Build history of the part. All positions in model axes, mm. A direction names the side the tool comes from. Give positions to 0.01 mm unless a question says otherwise; leave off trailing zeros. Order: outer loops, then holes, each group sorted by start corner. A loop starts at its lowest first (then second) coordinate and runs counter-clockwise, first axis right, second up. Notation, with made-up numbers: (10, 33.25) - (39, 33.25) arc R33 cw to (39, 68.25) - close; hole circle Ø4 at (51, 17.5). An arc over 180 degrees is marked (long way). Use a Markdown table: item, result.
from build123d import *

# Parameters (mm, degrees)
BASE_FLANGE1_DEPTH      = 45
EDGE_FLANGE1_DEPTH      = 606
EDGE_FLANGE1_BEND_DEPTH = 606
SKETCH11_R              = 12
CUT_EXTRUDE1_DEPTH      = 10
FILLET1_R               = 3
M5_CLEARANCE_HOLE1_D    = 5.8
M5_CLEARANCE_HOLE2_D    = 5.8


# Sheet-metal steps are written as plain solids
with BuildPart() as part:
    # Sketch1 → Base-Flange1 (new, symmetric)
    with BuildSketch(Plane.XY):
        with BuildLine():
            Line((-325, 0), (-309, 0))
            ThreePointArc((-309, 0), (-306.171572875, 1.171572875), (-305, 4))
            Line((-305, 4), (-305, 48))
            ThreePointArc((-305, 48), (-304.414213562, 49.414213562), (-303, 50))
            Line((-303, 50), (303, 50))
            ThreePointArc((303, 50), (304.414213562, 49.414213562), (305, 48))
            Line((305, 48), (305, 4))
            ThreePointArc((305, 4), (306.171572875, 1.171572875), (309, 0))
            Line((309, 0), (325, 0))
            Line((325, 0), (325, 2))
            Line((325, 2), (309, 2))
            ThreePointArc((309, 2), (307.585786438, 2.585786438), (307, 4))
            Line((307, 4), (307, 48))
            ThreePointArc((307, 48), (305.828427125, 50.828427125), (303, 52))
            Line((303, 52), (-303, 52))
            ThreePointArc((-303, 52), (-305.828427125, 50.828427125), (-307, 48))
            Line((-307, 48), (-307, 4))
            ThreePointArc((-307, 4), (-307.585786438, 2.585786438), (-309, 2))
            Line((-309, 2), (-325, 2))
            Line((-325, 2), (-325, 0))
        make_face()
    extrude(amount=BASE_FLANGE1_DEPTH, both=True)

    # Edge-Flange1 section (across the edge) → Edge-Flange1 (add)
    with BuildSketch(Plane(origin=(303, 52, -47), x_dir=(0, 0, 1), z_dir=(-1, 0, 0))):
        with BuildLine():
            Line((-2, 2), (-2, 18))
            Line((-2, 18), (0, 18))
            Line((0, 18), (0, 2))
            ThreePointArc((0, 2), (0.585786438, 0.585786438), (2, 0))
            Line((2, 0), (2, -2))
            ThreePointArc((2, -2), (-0.828427125, -0.828427125), (-2, 2))
        make_face()
    extrude(amount=EDGE_FLANGE1_DEPTH)

    # Edge-Flange1 section 2 (across the edge) → Edge-Flange1 bend (add)
    with BuildSketch(Plane(origin=(-303, 52, 47), x_dir=(0, 0, -1), z_dir=(1, 0, 0))):
        with BuildLine():
            Line((-2, 2), (-2, 18))
            Line((-2, 18), (0, 18))
            Line((0, 18), (0, 2))
            ThreePointArc((0, 2), (0.585786438, 0.585786438), (2, 0))
            Line((2, 0), (2, -2))
            ThreePointArc((2, -2), (-0.828427125, -0.828427125), (-2, 2))
        make_face()
    extrude(amount=EDGE_FLANGE1_BEND_DEPTH)

    # Sketch11 → Cut-Extrude1 (cut)
    with BuildSketch(Plane(origin=(0, 52, 0), x_dir=(1, 0, 0), z_dir=(0, 1, 0))):
        with Locations(Location((-65, 0, 0), (0, 0, 270))):
            Circle(SKETCH11_R)
        with Locations(Location((65, 0, 0), (0, 0, 270))):
            Circle(SKETCH11_R)
    extrude(amount=-CUT_EXTRUDE1_DEPTH, mode=Mode.SUBTRACT)

    # Fillet1
    fillet1_edges = [part.edges().sort_by_distance(p)[0] for p in [
        (-325, 1, -45),
        (325, 1, -45),
        (-325, 1, 45),
        (303, 70, -48),
        (-303, 70, -48),
        (325, 1, 45),
        (-303, 70, 48),
        (303, 70, 48),
    ]]
    fillet(fillet1_edges, radius=FILLET1_R)

    # M5 Clearance Hole1 (through all)
    with Locations(Plane(origin=(0, 2, 0), x_dir=(1, 0, 0), z_dir=(0, 1, 0))):
        with Locations((316.5, 27.5), (316.5, -27.5)):
            m5_clearance_hole1 = Hole(M5_CLEARANCE_HOLE1_D / 2)

    # Mirror1: M5 Clearance Hole1 across plane
    add(m5_clearance_hole1.mirror(Plane(origin=(0, 0, 0), x_dir=(0, 0, 1), z_dir=(1, 0, 0))), mode=Mode.SUBTRACT)

    # M5 Clearance Hole2 (through all)
    with Locations(Plane(origin=(0, 52, 0), x_dir=(1, 0, 0), z_dir=(0, 1, 0))):
        with Locations((-91, 0), (-65, 26), (-39, 0), (-65, -26)):
            m5_clearance_hole2 = Hole(M5_CLEARANCE_HOLE2_D / 2)

    # Mirror2: M5 Clearance Hole2 across plane
    add(m5_clearance_hole2.mirror(Plane(origin=(0, 0, 0), x_dir=(0, 0, 1), z_dir=(1, 0, 0))), mode=Mode.SUBTRACT)


solid = part.part
1) Slice it at C-C (y = 60.5). Write the cut outline in (x, z), and give its area (3 significant figures).
Computed:
| item | result |
|---|---|
| outline | (-303, -49) - (303, -49) - (303, -47) - (-303, -47) - close; (-303, 47) - (303, 47) - (303, 49) - (-303, 49) - close |
| area | 2,420 mm² |
2) Wall check: line 1 (Z direction, x = -157.5, y = 67.5); line 2 (X direction, y = 34, z = -28); line 3 (Z direction, x = 316.5, y = 1.05). Give the ranges that are in metal, low to high. Write a range as from..to.
Computed:
| item | result |
|---|---|
| line 1 | z = -49..-47, 47..49 |
| line 2 | x = -307..-305, 305..307 |
| line 3 | z = -45..-30.4, -24.6..24.6, 30.4..45 |
3) Pin check, flat tips, straight feed: P1, Ø9.5, axis at x = -316, y = 20, coming from the -Z side; P2, Ø3, axis at x = 0.5, z = -20, coming from the +Y side; P3, Ø13, axis at x = -314, z = 16.5, coming from the +Y side; P4, Ø1.5, axis at y = 47.5, z = -5, coming from the +X side. Stop position of each tip, or through.
Computed:
| item | result |
|---|---|
| P1 | passes through |
| P2 | stops at y = 52 |
| P3 | stops at y = 2.68 |
| P4 | stops at x = 307 |
4) Two-plate mould, pull along X, no slides. Class faces 6 (the flat face through (-306, 20, -45)), 7 (the flat face through (-4, 50, 1)), 8 (the flat face through (305, 26, 1)), 9 (the flat face through (-307, 26, 1)): +X half, -X half, draft (parallel to the pull), parting line (faces both ways), or undercut.
Computed:
| item | result |
|---|---|
| face 6 | draft |
| face 7 | undercut |
| face 8 | undercut |
| face 9 | -X half |
5) Tool access for faces 1 (the flat face through (307, 26, 1)), 2 (the flat face through (4, 62, -47)), 3 (the flat face through (-317, 2, 1)), 4 (the flat face through (4, 62, -49)), 5 (the flat face through (-305, 26, 1)): list every direction of +Z, -Z, +X, -X, +Y, -Y with a clear straight run to the whole face (end or side of a thin tool).
Computed:
| item | result |
|---|---|
| face 1 | +Z, -Z, +X, +Y |
| face 2 | +X, -X, +Y |
| face 3 | +Z, -Z, -X, +Y |
| face 4 | -Z, +X, -X, +Y, -Y |
| face 5 | +Z, -Z, -Y |
6) Slice it at B-B (x = 29.5). Write the cut outline in (y, z), and give its area (3 significant figures).
Computed:
| item | result |
|---|---|
| outline | (50, -45) arc R4 ccw to (54, -49) - (70, -49) - (70, -47) - (54, -47) arc R2 cw to (52, -45) - (52, 45) arc R2 cw to (54, 47) - (70, 47) - (70, 49) - (54, 49) arc R4 ccw to (50, 45) - close |
| area | 263 mm² |
7) Slice it at A-A (y = 14). Write the cut outline in (x, z).
Computed:
| item | result |
|---|---|
| outline | (-307, -45) - (-305, -45) - (-305, 45) - (-307, 45) - close; (305, -45) - (307, -45) - (307, 45) - (305, 45) - close |
